from build123d import *

# Parameters (mm, degrees)
SKETCH1_R           = 6
BOSS_EXTRUDE1_DEPTH = 2
BOSS_EXTRUDE2_DEPTH = 8
SKETCH3_R           = 5
BOSS_EXTRUDE3_DEPTH = 4
FILLET1_R           = 1


with BuildPart() as part:
    # Sketch1 → Boss-Extrude1 (new body)
    with BuildSketch(Plane(origin=(0, 0, 0), x_dir=(1, 0, 0), z_dir=(0, 1, 0))):
        with BuildLine():
            Line((1, 0), (19, 0))
            ThreePointArc((19, 0), (19.707106781, 0.292893219), (20, 1))
            Line((20, 1), (20, 19))
            ThreePointArc((20, 19), (19.707106781, 19.707106781), (19, 20))
            Line((19, 20), (1, 20))
            ThreePointArc((1, 20), (0.292893219, 19.707106781), (0, 19))
            Line((0, 19), (0, 1))
            ThreePointArc((0, 1), (0.292893219, 0.292893219), (1, 0))
        make_face()
        with Locations(Location((10, 10, 0), (0, 0, 270))):
            Circle(SKETCH1_R, mode=Mode.SUBTRACT)
    extrude(amount=BOSS_EXTRUDE1_DEPTH)

    # Sketch2 → Boss-Extrude2 (add)
    with BuildSketch(Plane(origin=(0, 0, 0), x_dir=(1, 0, 0), z_dir=(0, 1, 0))):
        with BuildLine():
            Line((2, 1), (18, 1))
            ThreePointArc((18, 1), (18.707106781, 1.292893219), (19, 2))
            Line((19, 2), (19, 18))
            ThreePointArc((19, 18), (18.707106781, 18.707106781), (18, 19))
            Line((18, 19), (2, 19))
            ThreePointArc((2, 19), (1.292893219, 18.707106781), (1, 18))
            Line((1, 18), (1, 2))
            ThreePointArc((1, 2), (1.292893219, 1.292893219), (2, 1))
        make_face()
    extrude(amount=-BOSS_EXTRUDE2_DEPTH)

    # Sketch3 → Boss-Extrude3 (add)
    with BuildSketch(Plane(origin=(0, 0, 0), x_dir=(1, 0, 0), z_dir=(0, 1, 0))):
        with Locations(Location((10, 10, 0), (0, 0, 270))):
            Circle(SKETCH3_R)
    extrude(amount=BOSS_EXTRUDE3_DEPTH)

    # Fillet1
    fillet1_edges = [part.edges().sort_by_distance(p)[0] for p in [
        (19.707106781, 2, -0.292893219),
        (20, 2, -10),
        (19.707106781, 2, -19.707106781),
        (10, 2, -20),
        (0.292893219, 2, -19.707106781),
        (0, 2, -10),
        (0.292893219, 2, -0.292893219),
        (10, 4, -15),
        (10, 2, 0),
    ]]
    fillet(fillet1_edges, radius=FILLET1_R)


solid = part.part
Here's how the part is built. I have some questions about the finished solid (model axes, mm). A direction names the side the tool comes from. Coordinates: 2 decimals unless noted, no trailing zeros. Loops run counter-clockwise (first coordinate to the right, second up) from the corner with the lowest first, then second, coordinate; pieces in that order, holes last. Notation, with made-up numbers: (-13.75, -23) -> (40.25, -23) arc R22 ccw to (40.25, -12) -> close; hole circle Ø3 at (-26.5, -10.75). An arc over 180 degrees is marked (long way). Use one line per item in the form item = value. Start each with the question number.
(1) If we section it at C-C (y = -1.75): Please give me the cut outline in (x, z), then the cut area to 3 significant figures.
(2) We'd pull the mould along Z, two halves only. Please class faces 1 (the face through (10, -4, -19)), 2 (the face through (1.285, -3.944, -1.301)), 3 (the face through (6, 0, -14)): pulls with the +Z half, pulls with the -Z half, needs draft (parallel to the pull), parting line crosses it, or undercut.
(3) If we section it at B-B (z = -10): Please give me the cut outline in (x, y).
(4) If we section it at D-D (x = 3): Please give me the cut outline in (y, z).
(5) If we section it at A-A (x = 10): Please give me the cut outline in (y, z).
(6) Please list where these lines run through material, in increasing order: line 1 along X through (y, z) = (0.65, -10); line 2 along X through (y, z) = (1.4, -10); line 3 along Z through (x, y) = (12.25, 1).
(7) Will these pins go through, and if not, where does the flat tip stop? pin 1 (6 mm diameter, centred on x = 9.5, y = -6.5, fed in from +Z); pin 2 (4 mm diameter, centred on x = 11, z = -16, fed in from +Y); pin 3 (1.5 mm diameter, centred on x = 8, y = -5, fed in from -Z).
(8) On a 3-axis mill with a long thin cutter (end or side, diameter ignored), from which of +Z, -Z, +X, -X, +Y, -Y can I reach the whole of each face in a straight line? I mean faces 4 (the face through (18.715, -3.944, -18.699)), 5 (the face through (19, -4, -10)), 6 (the face through (1, -4, -10)). Say none if no direction works.
Verdict:
q1.outline = (1, -18) arc R1 ccw to (2, -19) -> (18, -19) arc R1 ccw to (19, -18) -> (19, -2) arc R1 ccw to (18, -1) -> (2, -1) arc R1 ccw to (1, -2) -> close
q1.area = 323 mm²
q2.face_1 = pulls with the -Z half
q2.face_2 = pulls with the +Z half
q2.face_3 = undercut
q3.outline = (0, 0) -> (1, 0) -> (1, -8) -> (19, -8) -> (19, 0) -> (20, 0) -> (20, 1) arc R1 ccw to (19, 2) -> (16, 2) -> (16, 0) -> (15, 0) -> (15, 3) arc R1 ccw to (14, 4) -> (6, 4) arc R1 ccw to (5, 3) -> (5, 0) -> (4, 0) -> (4, 2) -> (1, 2) arc R1 ccw to (0, 1) -> close
q4.outline = (-8, -19) -> (0, -19) -> (0, -20) -> (1, -20) arc R1 ccw to (2, -19) -> (2, -1) arc R1 ccw to (1, 0) -> (0, 0) -> (0, -1) -> (-8, -1) -> close
q5.outline = (-8, -19) -> (0, -19) -> (0, -20) -> (1, -20) arc R1 ccw to (2, -19) -> (2, -16) -> (0, -16) -> (0, -15) -> (3, -15) arc R1 ccw to (4, -14) -> (4, -6) arc R1 ccw to (3, -5) -> (0, -5) -> (0, -4) -> (2, -4) -> (2, -1) arc R1 ccw to (1, 0) -> (0, 0) -> (0, -1) -> (-8, -1) -> close
q6.line_1 = 0 to 4, 5 to 15, 16 to 20
q6.line_2 = 0.08 to 4, 5 to 15, 16 to 19.92
q6.line_3 = -20 to -15.56, -14.47 to -5.53, -4.44 to 0
q7.pin_1 = -1
q7.pin_2 = 4
q7.pin_3 = -19
q8.face_4 = -Z, +X, -Y
q8.face_5 = +Z, -Z, +X, -Y
q8.face_6 = +Z, -Z, -X, -Y
